from build123d import *

# Parameters (mm, degrees)
SKETCH_R           = 66.6
PAD_DEPTH          = 1250
PAD001_DEPTH       = 3.185
POLARPATTERN_COUNT = 3


with BuildPart() as part:
    # Sketch → Pad (new body)
    with BuildSketch(Plane.XY):
        Circle(SKETCH_R)
    extrude(amount=PAD_DEPTH)

    # Sketch001 → Revolution (revolve)
    with BuildSketch(Plane.XZ):
        with BuildLine():
            Line((0, 1500), (0, 1250))
            Line((0, 1250), (-66.6, 1250))
            add(Edge.make_bspline(
                [(0, 1500), (-35, 1450), (-66.6, 1375), (-66.6, 1250)],
                knots=[0, 0, 0, 0, 1, 1, 1, 1], degree=3))
        make_face()
    revolve(axis=Axis((0, 0, 0), (0, 0, 1)))

    # Sketch002 → Pad001 (join, symmetric)
    with BuildSketch(Plane.XZ):
        Polygon((66.6, 240), (186.6, 60), (186.6, 0), (66.6, 0), (0, 0), (0, 240), align=None)
    pad001 = extrude(amount=PAD001_DEPTH, both=True)

    # PolarPattern: Pad001 ×3 about axis
    polarpattern_axis = Axis((0, 0, 0), (0, 0, 1))
    for i in range(1, POLARPATTERN_COUNT):
        add(pad001.rotate(polarpattern_axis, i * 360 / POLARPATTERN_COUNT))


solid = part.part
Here's how the part is built. I have some questions about the finished solid (model axes, mm). A direction names the side the tool comes from. Round coordinates to 2 decimals unless told otherwise and drop trailing zeros. Order: outer loops, then holes, each group sorted by start corner. A loop starts at its lowest first (then second) coordinate and runs counter-clockwise, first axis right, second up. Notation, with made-up numbers: (-1, 82.5) -> (48, 82.5) arc R22 cw to (48, 111.5) -> close; hole circle Ø6 at (1, 55). An arc over 180 degrees is marked (long way). Use CSV: the item, a comma, the result in double quotes.
1. I want a section at D-D on z = 331.5. List the corners of the cut face in (x, y) for me.
Recorded:
outline,"circle Ø133.2 at (0, 0)"
2. I need wall thicknesses on line 1 along Y through (x, z) = (31, 589); line 2 along Z through (x, y) = (-24.5, -34.5); line 3 along Y through (x, z) = (8.5, 117.5). Which ranges of each line are inside material? Lowest first, please.
Recorded:
line 1,"y = -58.95 to 58.95"
line 2,"z = 0 to 1415.92"
line 3,"y = -66.06 to 66.06"
3. Which directions (+Z, -Z, +X, -X, +Y, -Y) give clear straight access to the entire face, cutting with the end or side of a thin tool? Please do faces 1 (the face through (-54.27, -100.37, 95.01)), 2 (the face through (-7, -11, 0)), 3 (the face through (114, 3.185, 95)), 4 (the face through (-59.79, 97.19, 95.01)).
Recorded:
face 1,"+Z, -Z, -Y"
face 2,"-Z, +X, -X, +Y, -Y"
face 3,"+Z, -Z, +X, +Y"
face 4,"+Z, -Z, -X"
4. Thinking about a two-plate mould opening in Y: for faces 5 (the face through (114, -3.185, 95)), 6 (the face through (-59.79, -97.19, 95.01)), 7 (the face through (-62.841, 108.934, 151.26)), which applies, pulls with the +Y half, pulls with the -Y half, needs draft (parallel to the pull), parting line crosses it, or undercut?
Recorded:
face 5,"pulls with the -Y half"
face 6,"undercut"
face 7,"pulls with the +Y half"
5. I want a section at A-A on z = 105. List the corners of the cut face in (x, y) for me (3 decimals).
Recorded:
outline,"(-81.058, -134.027) -> (-75.542, -137.212) -> (-30.504, -59.204) arc R66.6 ccw to (66.524, -3.185) -> (156.6, -3.185) -> (156.6, 3.185) -> (66.524, 3.185) arc R66.6 ccw to (-30.504, 59.204) -> (-75.542, 137.212) -> (-81.058, 134.027) -> (-36.02, 56.019) arc R66.6 ccw to (-36.02, -56.019) -> close"
6. I want a section at C-C on x = 159. List the corners of the cut face in (y, z) for me (3 decimals), and give its area (3 significant figures).
Recorded:
outline,"(-3.185, 0) -> (3.185, 0) -> (3.185, 101.4) -> (-3.185, 101.4) -> close"
area,"646 mm2"
7. I want a section at B-B on y = 134. List the corners of the cut face in (x, z) for me, and give its area (3 significant figures).
Recorded:
outline,"(-81.04, 0) -> (-73.69, 0) -> (-73.69, 110.56) -> (-81.04, 105.05) -> close"
area,"793 mm2"
8. I'm going to push flat-ended pins straight in: P1, Ø10, axis at x = -35.5, z = 652.5, coming from the -Y side; P2, Ø0.5, axis at x = -32.5, y = 59, coming from the +Z side; P3, Ø1, axis at x = -42, z = 457.5, coming from the -Y side. Where does each tip first touch, or does it pass through?
Recorded:
P1,"stops at y = -59.21"
P2,"stops at z = 239.26"
P3,"stops at y = -52.09"
